```python
from build123d import *

# Parameters (mm, degrees)
SKETCH1_W           = 70
SKETCH1_H           = 12
BOSS_EXTRUDE2_DEPTH = 12


with BuildPart() as part:
    # Sketch1 → Boss-Extrude2 (new body)
    with BuildSketch(Plane.XY):
        Polygon((280, 1000), (350, 1000), (350, 565), (338, 565), (338, 475), (350, 475), (350, 370), (338, 370), (338, 280), (350, 280), (350, 175), (338, 175), (338, 85), (350, 85), (350, 0), (280, 0), (280, 12), (210, 12), (210, 0), (140, 0), (140, 12), (70, 12), (70, 0), (0, 0), (0, 720), (12, 720), (12, 790), (0, 790), (0, 860), (12, 860), (12, 930), (0, 930), (0, 1000), (70, 1000), (70, 988), (140, 988), (140, 1000), (210, 1000), (210, 988), (280, 988), align=None)
        with Locations((105, 656)):
            Rectangle(SKETCH1_W, SKETCH1_H, mode=Mode.SUBTRACT)
        with Locations((245, 656)):
            Rectangle(SKETCH1_W, SKETCH1_H, mode=Mode.SUBTRACT)
    extrude(amount=BOSS_EXTRUDE2_DEPTH)


solid = part.part
```
Build history of the part. All positions in model axes, mm. Coordinates: 2 decimals unless noted, no trailing zeros. Write each loop counter-clockwise with the first axis right and the second up, starting at its lowest first coordinate (ties: lowest second). Pieces come first, ordered by that corner, then holes.
1. Band-saw the part on B-B, the plane z = 7. Give the number of separate pieces and of enclosed holes in the cut face, and give its area (3 significant figures).
Answer block:
separate pieces: 1
enclosed holes: 2
area: 340,000 mm2
2. Band-saw the part on A-A, the plane x = 88. Give the cut face in (y, z).
Answer block:
outline: (12, 0) - (650, 0) - (650, 12) - (12, 12) - close; (662, 0) - (988, 0) - (988, 12) - (662, 12) - close
3. Band-saw the part on C-C, the plane y = 497. Give the cut face in (x, z).
Answer block:
outline: (0, 0) - (338, 0) - (338, 12) - (0, 12) - close
4. Drop flat-ended pins along their axis: pin 1 (3 mm diameter, centred on x = 87, z = 10, fed in from +Y); pin 2 (3.5 mm diameter, centred on x = 235.5, z = 7.5, fed in from -Y); pin 3 (6 mm diameter, centred on y = 896.5, z = 7, fed in from -X). Give the stop position or say it passes through.
Answer block:
pin 1: stops at y = 988
pin 2: stops at y = 12
pin 3: stops at x = 12
5. Drill centre lines: probe 1 along Y at (x, z) = (98, 5.75); probe 2 along X at (y, z) = (781, 8.75). Where is each one in solid material? Low to high.
Answer block:
probe 1: y = 12 to 650, 662 to 988
probe 2: x = 12 to 350
